Geometry: see drawing. Coordinates: mm, zero at the bounding-box minimum. A direction names the side the tool comes from. Give positions to 0.01 mm unless a question says otherwise; leave off trailing zeros. Write each loop counter-clockwise with the first axis right and the second up, starting at its lowest first coordinate (ties: lowest second). Pieces come first, ordered by that corner, then holes. Notation, with made-up numbers: (62, 4) - (112, 4) arc R22 ccw to (112, 29) - close; hole circle Ø11 at (69.5, -27). An arc over 180 degrees is marked (long way). Answer as CSV lines item,"result". Start each with the question number.
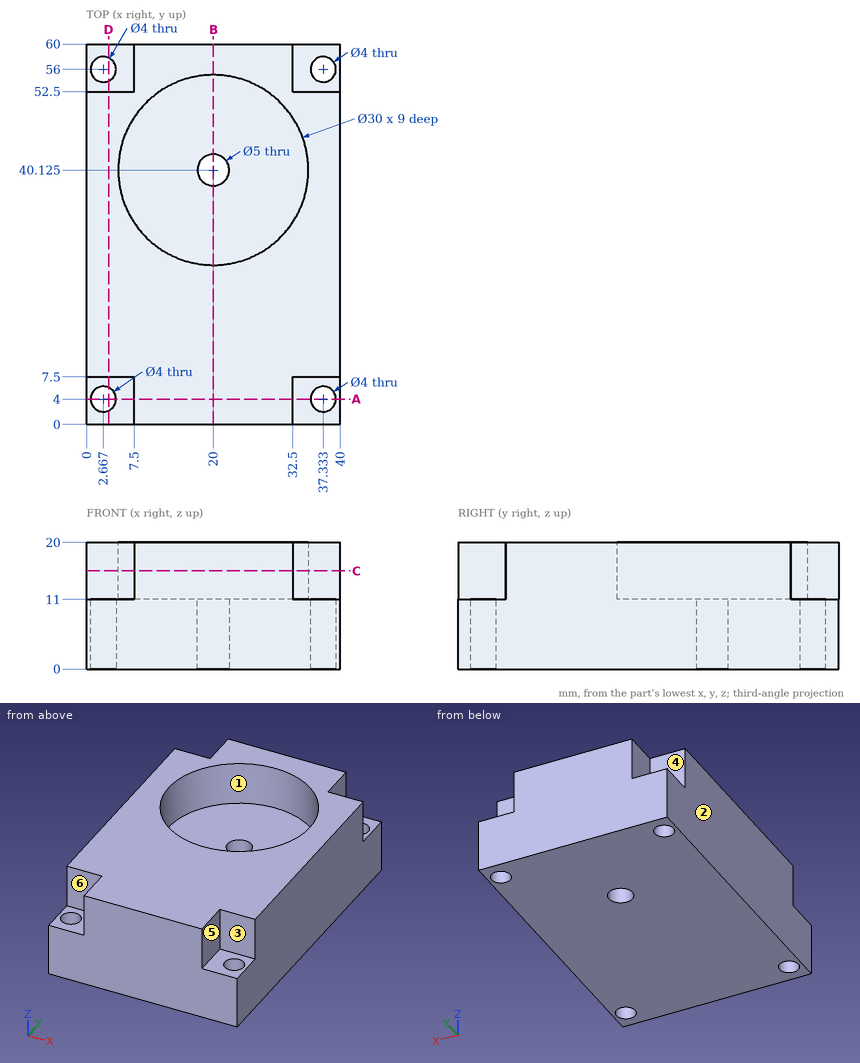
1) Material intervals for line 1 (Y direction, x = 20, z = 14.75) (1 decimal); line 2 (Y direction, x = 20, z = 6) (1 decimal); line 3 (Y direction, x = 38.5, z = 10.25) (1 decimal), sorted ascending. Write a range as from..to.
2) Cut plane A-A on y = 4. Output: boundary loops of the cut face in (x, z).
3) Contact query for flat-ended pins moving along their axis: P1, Ø24, axis at x = 20, y = 40.125, coming from the +Z side; P2, Ø4, axis at x = 35.5, z = 16.5, coming from the -Y side; P3, Ø8, axis at x = 37, z = 17, coming from the +Y side; P4, Ø3, axis at x = 20, y = 40.125, coming from the -Z side. Output: stop coordinate, or through.
4) Cut plane B-B on x = 20. Output: boundary loops of the cut face in (y, z) (1 decimal), and give its area (3 significant figures).
5) Pull-direction query (X, two-part tool) for the marked faces 1, 2 and 3; classes: +X half, -X half, draft (parallel to the pull), parting line (faces both ways), or undercut.
6) Reachability of the marked faces 4, 5 and 6 from +Z, -Z, +X, -X, +Y, -Y: full face, straight path, thin tool, end or side. Return the list, or none.
7) Cut plane D-D on x = 3.5. Output: boundary loops of the cut face in (y, z).
8) Cut plane C-C on z = 15.5. Output: boundary loops of the cut face in (x, y) (1 decimal).
Numbers:
1,line 1,"y = 0..25.1, 55.1..60"
1,line 2,"y = 0..37.6, 42.6..60"
1,line 3,"y = 0..2.4, 5.6..54.4, 57.6..60"
2,outline,"(0, 0) - (0.67, 0) - (0.67, 11) - (0, 11) - close; (4.67, 0) - (35.33, 0) - (35.33, 11) - (32.5, 11) - (32.5, 20) - (7.5, 20) - (7.5, 11) - (4.67, 11) - close; (39.33, 0) - (40, 0) - (40, 11) - (39.33, 11) - close"
3,P1,"stops at z = 11"
3,P2,"stops at y = 7.5"
3,P3,"stops at y = 52.5"
3,P4,"passes through"
4,outline,"(0, 0) - (37.6, 0) - (37.6, 11) - (25.1, 11) - (25.1, 20) - (0, 20) - close; (42.6, 0) - (60, 0) - (60, 20) - (55.1, 20) - (55.1, 11) - (42.6, 11) - close"
4,area,"875 mm²"
5,face 1,"undercut"
5,face 2,"-X half"
5,face 3,"draft"
6,face 4,"+Z, -X, +Y"
6,face 5,"+Z, +X, -Y"
6,face 6,"+Z, -X, -Y"
7,outline,"(0, 0) - (2.18, 0) - (2.18, 11) - (0, 11) - close; (5.82, 0) - (54.18, 0) - (54.18, 11) - (52.5, 11) - (52.5, 20) - (7.5, 20) - (7.5, 11) - (5.82, 11) - close; (57.82, 0) - (60, 0) - (60, 11) - (57.82, 11) - close"
8,outline,"(0, 7.5) - (7.5, 7.5) - (7.5, 0) - (32.5, 0) - (32.5, 7.5) - (40, 7.5) - (40, 52.5) - (32.5, 52.5) - (32.5, 60) - (7.5, 60) - (7.5, 52.5) - (0, 52.5) - close; hole circle Ø30 at (20, 40.1)"
